Autodesk Fusion 360 part; units mm, degrees
sketch "Sketch1" plane through (0, 0, 0) normal (0, 1, 0) x (1, 0, 0)
  line L0 (0, 0) -> (20, 0)
  line L1 (20, 0) -> (20, -25.4)
  line L2 (20, -25.4) -> (0, -25.4)
  line L3 (0, -25.4) -> (0, 0)
  line L4 (10, -25.4) -> (10, 0) construction
  line L5 (16.5, -16.4528) -> (16.5, -8.9472)
  line L6 (16.5, -8.9472) -> (10, -5.1944)
  line L7 (10, -5.1944) -> (3.5, -8.9472)
  line L8 (3.5, -8.9472) -> (3.5, -16.4528)
  line L9 (3.5, -16.4528) -> (10, -20.2056)
  line L10 (10, -20.2056) -> (16.5, -16.4528)
  circle A0 centre (10, -12.7) radius 4.2
  line L11 (16.5, -16.4528) -> (16.5, -25.4)
  line L12 (3.5, -16.4528) -> (3.5, -25.4)
  point P0 (10, -12.7)
  dimension "d1" = 20
  dimension "d2" = 25.4
  dimension "d3" = 13
  dimension "d4" = 8.4
extrude "Extrude1" add sketch "Sketch1" along normal blind 70 contours L0 L1 L2 L3 L5 L6 L7 L8 L11 L12 | L2 L9 L10 L11 L12 | L5 L6 L7 L8 L9 L10 | A0
extrude "Extrude5" cut sketch "Sketch1" along normal blind 25 contours A0
extrude "Extrude2" cut sketch "Sketch1" along normal blind 7 from surface at 6 contours L2 L9 L10 L11 L12 | L5 L6 L7 L8 L9 L10
sketch "Sketch2" plane through (0, 0, 0) normal (-1, 0, 0) x (0, -1, 0)
  line L0 (0, 0) -> (0, 25.4)
  line L1 (0, 25.4) -> (-70, 25.4)
  line L2 (-70, 25.4) -> (-70, 0)
  line L3 (-70, 0) -> (0, 0)
  line L4 (-70, 12.7) -> (0, 12.7) construction
  line L5 (-58, 5.1944) -> (-51.5, 8.9472)
  line L6 (-51.5, 8.9472) -> (-51.5, 16.4528)
  line L7 (-51.5, 16.4528) -> (-58, 20.2056)
  line L8 (-58, 20.2056) -> (-64.5, 16.4528)
  line L9 (-64.5, 16.4528) -> (-64.5, 8.9472)
  line L10 (-64.5, 8.9472) -> (-58, 5.1944)
  circle A0 centre (-58, 12.7) radius 4.2
  line L11 (-64.5, 16.4528) -> (-64.5, 25.4)
  line L12 (-51.5, 16.4528) -> (-51.5, 25.4)
  circle A1 centre (-38, 12.7) radius 4.2
  line L13 (-31.5, 8.9472) -> (-31.5, 16.4528)
  line L14 (-31.5, 16.4528) -> (-38, 20.2056)
  line L15 (-38, 20.2056) -> (-44.5, 16.4528)
  line L16 (-44.5, 16.4528) -> (-44.5, 8.9472)
  line L17 (-44.5, 8.9472) -> (-38, 5.1944)
  line L18 (-38, 5.1944) -> (-31.5, 8.9472)
  line L19 (-44.5, 16.4528) -> (-44.5, 25.4)
  line L20 (-31.5, 16.4528) -> (-31.5, 25.4)
  point P0 (-58, 12.7)
  point P1 (-38, 12.7)
  dimension "d11" = 12
  dimension "d12" = 13
  dimension "d13" = 8.4
  dimension "d20" = 20
extrude "Extrude3" cut sketch "Sketch2" against normal blind 24 contours A0 | A1
extrude "Extrude4" cut sketch "Sketch2" against normal blind 7 from surface at -6.5 contours L1 L14 L15 L19 L20 | L13 L14 L15 L16 L17 L18 | L1 L7 L8 L11 L12 | L5 L6 L7 L8 L9 L10
chamfer "Chamfer1" distance 0.4 angle 45 29 edges at (0, 70, 12.7) (20, 70, 12.7) (20, 0, 12.7) (0, 0, 12.7) (0, 35, 0) (0, 35, 25.4) (10, 0, 0) (10, 0, 25.4) (20, 35, 25.4) (10, 70, 25.4) (10, 64.5, 25.4) (6.5, 58, 25.4) (13.5, 58, 25.4) (10, 51.5, 25.4) (10, 13, 25.4) (16.5, 9.5, 25.4) (10, 6, 25.4) (3.5, 9.5, 25.4) (0, 61.9158, 14.2188) (10, 70, 0) (20, 61.9158, 11.1812) (20, 35, 0) (10, 44.5, 25.4) (13.5, 38, 25.4) (10, 31.5, 25.4) (6.5, 38, 25.4) (20, 41.9158, 11.1812) (6.0842, 0, 14.2188) (0, 41.9158, 14.2188)
CAD build for the part. Positions are in the model's coordinates, mm. A direction names the side the tool comes from. Give positions to 0.01 mm unless a question says otherwise; leave off trailing zeros. Order: outer loops, then holes, each group sorted by start corner. A loop starts at its lowest first (then second) coordinate and runs counter-clockwise, first axis right, second up.
(1) Mould opens along X. For faces 1 (the flat face through (20, 35, 18)), 2 (the flat face through (13.5, 38.1, 17.4)), 3 (the flat face through (6.8, 9.45, 7.04)), 4 (the flat face through (14.4, 34.5, 25.4)) say: released by +X, released by -X, zero draft, split by the parting line, or undercut.
(2) Tool access for faces 5 (the flat face through (13.3, 9.5, 7.1)), 6 (the cylindrical face through (9.09, 18.92, 8.6)), 7 (the cylindrical face through (16.507, 33.994, 13.962)): list every direction of +Z, -Z, +X, -X, +Y, -Y with a clear straight run to the whole face (end or side of a thin tool).
(3) Saw through at D-D, the plane z = 12.7. State how many separate pieces and enclosed holes the cut face has, then the cut area to 3 significant figures.
(4) Saw through at A-A, the plane x = 1.5. Give the cut face in (y, z).
(5) Drill centre lines: L1, parallel to Y at x = 7, z = 18; L2, parallel to Y at x = 9.25, z = 11; L3, parallel to X at y = 4.3, z = 12.7. Where is each one in solid material? Low to high.
(6) Saw through at C-C, the plane z = 7. Give the cut face in (x, y).
(7) Saw through at B-B, the plane y = 24. Give the cut face in (x, z), then the cut area to 3 significant figures.
Results found:
1. face 1: released by +X
1. face 2: undercut
1. face 3: undercut
1. face 4: zero draft
2. face 5: +Z
2. face 6: -Y
2. face 7: +X, -X
3. separate pieces: 3
3. enclosed holes: 0
3. area: 756 mm2
4. outline: (0, 0.4) - (0.4, 0) - (69.6, 0) - (70, 0.4) - (70, 25) - (69.6, 25.4) - (0.4, 25.4) - (0, 25) - close; hole circle Ø8.4 at (38, 12.7); hole circle Ø8.4 at (58, 12.7)
5. L1: y = 0 to 6, 13 to 31.5, 44.5 to 51.5, 64.5 to 70
5. L2: y = 25 to 31.5, 44.5 to 51.5, 64.5 to 70
5. L3: x = 0 to 5.8, 14.2 to 20
6. outline: (0, 0.4) - (0.4, 0) - (19.6, 0) - (20, 0.4) - (20, 69.6) - (19.6, 70) - (0.4, 70) - (0, 69.6) - close; hole (6.5, 34.87) - (13.5, 34.87) - (13.5, 41.13) - (6.5, 41.13) - close; hole (6.5, 54.87) - (13.5, 54.87) - (13.5, 61.13) - (6.5, 61.13) - close; hole (6.87, 6) - (13.13, 6) - (13.13, 13) - (6.87, 13) - close
7. outline: (0, 0.4) - (0.4, 0) - (19.6, 0) - (20, 0.4) - (20, 25) - (19.6, 25.4) - (0.4, 25.4) - (0, 25) - close; hole circle Ø8.4 at (10, 12.7)
7. area: 452 mm2
